Could you check a few things on this model? Use its own coordinates, in mm. A direction names the side the tool comes from. Coordinates: 2 decimals unless noted, no trailing zeros. Loops run counter-clockwise (first coordinate to the right, second up) from the corner with the lowest first, then second, coordinate; pieces in that order, holes last.
1) For faces 4 (the face through (20, 19, -15)), 5 (the face through (69, 14, -15)), 6 (the face through (3, 7.1, -5.46)), which set-ups out of +Z, -Z, +X, -X, +Y, -Y let a thin tool reach every point of the face, with its end or its side?
2) Will these pins go through, and if not, where does the flat tip stop? P1, Ø6, axis at y = 27.5, z = -24, coming from the -X side; P2, Ø2, axis at x = 21.5, z = -16, coming from the +Y side; P3, Ø9, axis at x = -5.5, z = -20.5, coming from the +Y side; P4, Ø15, axis at y = 27.5, z = -18, coming from the +X side.
3) Imagine slicing it at B-B on z = -14. Please give me the cut outline in (x, y), plus the area to 3 significant figures.
4) Thinking about a two-plate mould opening in X: for faces 1 (the face through (60, 19, -15)), 2 (the face through (88.43, 7.1, -9.62)), 3 (the face through (40, 45, -15)), which applies, released by +X, released by -X, zero draft, split by the parting line, or undercut?
5) Imagine slicing it at D-D on x = 83. Please give me the cut outline in (y, z), plus the area to 3 significant figures.
6) If I drill on line 1 along X through (y, z) = (9.75, -15); line 2 along Y through (x, z) = (34, -15); line 3 along Z through (x, y) = (34, 29), over which ranges is the centre line in solid material (lowest first)?
7) Imagine slicing it at C-C on y = 22. Please give me the cut outline in (x, z).
8) Imagine slicing it at A-A on y = 11.5. Please give me the cut outline in (x, z), plus the area to 3 significant figures.
```python
from build123d import *

# Parameters (mm, degrees)
SALIENTE_EXTRUIR1_DEPTH = 14
CROQUIS2_W              = 40
CROQUIS2_H              = 30
SALIENTE_EXTRUIR2_DEPTH = 16
CROQUIS3_R              = 15
SALIENTE_EXTRUIR4_DEPTH = 40
CROQUIS6_R              = 10
CORTAR_EXTRUIR1_DEPTH   = 96
CROQUIS8_R              = 10
CORTAR_EXTRUIR2_DEPTH   = 96
CROQUIS11_R             = 10
CORTAR_EXTRUIR3_DEPTH   = 96


with BuildPart() as part:
    # Croquis1 → Saliente-Extruir1 (new body)
    with BuildSketch(Plane(origin=(0, 0, 0), x_dir=(1, 0, 0), z_dir=(0, 1, 0))):
        with BuildLine():
            Line((0, 0), (80, 0))
            ThreePointArc((80, 0), (95, 15), (80, 30))
            Line((80, 30), (0, 30))
            ThreePointArc((0, 30), (-15, 15), (0, 0))
        make_face()
    extrude(amount=SALIENTE_EXTRUIR1_DEPTH)

    # Croquis2 → Saliente-Extruir2 (add)
    with BuildSketch(Plane(origin=(0, 14, 0), x_dir=(1, 0, 0), z_dir=(0, 1, 0))):
        with Locations((40, 15)):
            Rectangle(CROQUIS2_W, CROQUIS2_H)
    extrude(amount=SALIENTE_EXTRUIR2_DEPTH)

    # Croquis3 → Saliente-Extruir4 (add)
    with BuildSketch(Plane.ZY.offset(-20)):
        with Locations((-15, 30)):
            Circle(CROQUIS3_R)
    extrude(amount=-SALIENTE_EXTRUIR4_DEPTH)

    # Croquis6 → Cortar-Extruir1 (cut)
    with BuildSketch(Plane.ZY.offset(-20)):
        with Locations((-15, 29.5)):
            Circle(CROQUIS6_R)
    extrude(amount=-CORTAR_EXTRUIR1_DEPTH, mode=Mode.SUBTRACT)

    # Croquis8 → Cortar-Extruir2 (cut)
    with BuildSketch(Plane(origin=(0, 14, 0), x_dir=(1, 0, 0), z_dir=(0, 1, 0))):
        with Locations(Location((0, 15, 0), (0, 0, 270))):
            Circle(CROQUIS8_R)
    extrude(amount=-CORTAR_EXTRUIR2_DEPTH, mode=Mode.SUBTRACT)

    # Croquis11 → Cortar-Extruir3 (cut)
    with BuildSketch(Plane(origin=(0, 14, 0), x_dir=(1, 0, 0), z_dir=(0, 1, 0))):
        with Locations(Location((80, 15, 0), (0, 0, 270))):
            Circle(CROQUIS11_R)
    extrude(amount=-CORTAR_EXTRUIR3_DEPTH, mode=Mode.SUBTRACT)


solid = part.part
```
Filled in:
1. face 4: +Z, -Z, -X, +Y
1. face 5: +Z, -Z, +X, +Y
1. face 6: +Y, -Y
2. P1: stops at x = 20
2. P2: stops at y = 45
2. P3: stops at y = 14
2. P4: stops at x = 60
3. outline: (-14.97, 0) - (-9.95, 0) - (-9.95, 14) - (-14.97, 14) - close; (9.95, 0) - (70.05, 0) - (70.05, 14) - (60, 14) - (60, 19.55) - (20, 19.55) - (20, 14) - (9.95, 14) - close; (20, 39.45) - (60, 39.45) - (60, 44.97) - (20, 44.97) - close; (89.95, 0) - (94.97, 0) - (94.97, 14) - (89.95, 14) - close
3. area: 1,420 mm2
4. face 1: released by +X
4. face 2: undercut
4. face 3: zero draft
5. outline: (0, -29.7) - (14, -29.7) - (14, -24.54) - (0, -24.54) - close; (0, -5.46) - (14, -5.46) - (14, -0.3) - (0, -0.3) - close
5. area: 144 mm2
6. line 1: x = -15 to -10, 10 to 70, 90 to 95
6. line 2: y = 0 to 19.5, 39.5 to 45
6. line 3: z = -30 to -24.99, -5.01 to 0
7. outline: (20, -30) - (60, -30) - (60, -21.61) - (20, -21.61) - close; (20, -8.39) - (60, -8.39) - (60, 0) - (20, 0) - close
8. outline: (0, -30) - (80, -30) arc R15 ccw to (80, 0) - (0, 0) arc R15 ccw to start; hole circle Ø20 at (0, -15); hole circle Ø20 at (80, -15)
8. area: 2,480 mm2
